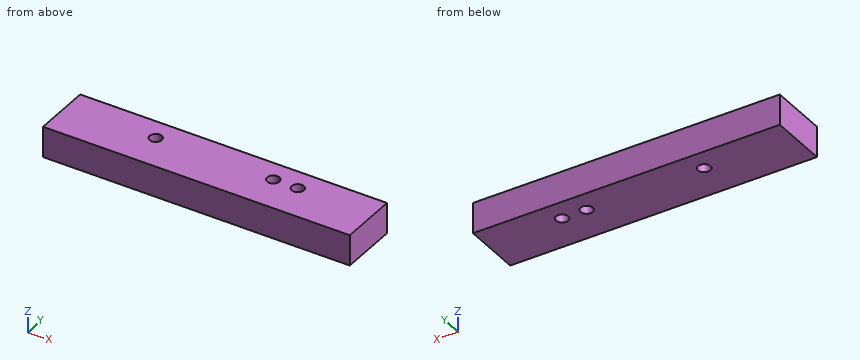
from build123d import *

# Parameters (mm, degrees)
SKETCH1_W           = 50
SKETCH1_H           = 5
BOSS_EXTRUDE1_DEPTH = 9.5
CUT_EXTRUDE1_REACH  = 35.869
SKETCH2_R           = 1


with BuildPart() as part:
    # Sketch1 → Boss-Extrude1 (new body)
    with BuildSketch(Plane(origin=(0, 10, 0), x_dir=(1, 0, 0), z_dir=(0, 1, 0))):
        with Locations((2.237632925, -48.5)):
            Rectangle(SKETCH1_W, SKETCH1_H)
    extrude(amount=BOSS_EXTRUDE1_DEPTH)

    # Sketch2 → Cut-Extrude1 (cut, up to next)
    with BuildSketch(Plane(origin=(0, 0, 46), x_dir=(-1, 0, 0), z_dir=(0, 0, -1)), mode=Mode.PRIVATE) as cut_extrude1_sk1:
        with Locations((-14.942868758, 16)):
            Circle(SKETCH2_R)
    cut_extrude1_tool1 = extrude(cut_extrude1_sk1.sketch, amount=-CUT_EXTRUDE1_REACH, mode=Mode.PRIVATE) & part.part
    # Sketch2 → Cut-Extrude1 (cut, up to next)
    with BuildSketch(Plane(origin=(0, 0, 46), x_dir=(-1, 0, 0), z_dir=(0, 0, -1)), mode=Mode.PRIVATE) as cut_extrude1_sk2:
        with Locations((8.213561031, 16)):
            Circle(SKETCH2_R)
    cut_extrude1_tool2 = extrude(cut_extrude1_sk2.sketch, amount=-CUT_EXTRUDE1_REACH, mode=Mode.PRIVATE) & part.part
    # Sketch2 → Cut-Extrude1 (cut, up to next)
    with BuildSketch(Plane(origin=(0, 0, 46), x_dir=(-1, 0, 0), z_dir=(0, 0, -1)), mode=Mode.PRIVATE) as cut_extrude1_sk3:
        with Locations((-10.942868758, 16)):
            Circle(SKETCH2_R)
    cut_extrude1_tool3 = extrude(cut_extrude1_sk3.sketch, amount=-CUT_EXTRUDE1_REACH, mode=Mode.PRIVATE) & part.part
    add(cut_extrude1_tool1.solids().sort_by_distance((14.942869, 16, 46))[0], mode=Mode.SUBTRACT)
    add(cut_extrude1_tool2.solids().sort_by_distance((-8.213561, 16, 46))[0], mode=Mode.SUBTRACT)
    add(cut_extrude1_tool3.solids().sort_by_distance((10.942869, 16, 46))[0], mode=Mode.SUBTRACT)


solid = part.part
Can you work these out from the model? Positions are in its coordinate system, mm. Coordinates: 2 decimals unless noted, no trailing zeros. Loops run counter-clockwise (first coordinate to the right, second up) from the corner with the lowest first, then second, coordinate; pieces in that order, holes last. Notation, with made-up numbers: M 72.25,-10 L 119.25,-10 A16 ccw 119.25,7 Z; hole C 7.5,14.25 d9. An arc over 180 degrees is marked long. Return JSON: item names as keys, results as strings. Group by question number.
Item 1: Imagine slicing it at A-A (z = 50.5). Please give me the cut outline in (x, y), and give its area (3 significant figures).
Item 2: If I drill on L1, parallel to Y at x = -8, z = 47.25; L2, parallel to Y at x = 15.5, z = 46.4, over which ranges is the centre line in solid material (lowest first)? Write a range as from..to.
Item 3: Imagine slicing it at B-B (y = 16.5). Please give me the cut outline in (x, z).
Verdict:
{
 "1": {"outline": "M -22.76,10 L 27.24,10 L 27.24,19.5 L -22.76,19.5 Z; hole C -8.21,16 d2; hole C 10.94,16 d2; hole C 14.94,16 d2", "area": "466 mm^2"},
 "2": {"L1": "y = 10..15.02, 16.98..19.5", "L2": "y = 10..15.17, 16.83..19.5"},
 "3": {"outline": "M -22.76,46 L -9.08,46 L -9.08,51 L -22.76,51 Z; M -7.35,46 L 10.08,46 L 10.08,51 L -7.35,51 Z; M 11.81,46 L 14.08,46 L 14.08,51 L 11.81,51 Z; M 15.81,46 L 27.24,46 L 27.24,51 L 15.81,51 Z"}
}
